```python
from build123d import *

# Parameters (mm, degrees)
SKETCH1_W             = 82.55
SKETCH1_H             = 57.15
BOSS_EXTRUDE1_DEPTH   = 3.175
CUT_EXTRUDE5_DEPTH    = 10
F_8_CLEARANCE_HOLE1_D = 4.4958
F_4_40_TAPPED_HOLE1_D = 2.2606


with BuildPart() as part:
    # Sketch1 → Boss-Extrude1 (new body)
    with BuildSketch(Plane(origin=(0, 0, 0), x_dir=(1, 0, 0), z_dir=(0, 1, 0))):
        Rectangle(SKETCH1_W, SKETCH1_H)
    extrude(amount=BOSS_EXTRUDE1_DEPTH)

    # Sketch2 → Cut-Extrude5 (cut)
    with BuildSketch(Plane.XZ):
        with BuildLine():
            Line((8.5, 1.825), (8.5, 0.175))
            ThreePointArc((8.5, 0.175), (9.42993597, -2.07006403), (11.675, -3))
            Line((11.675, -3), (15.325, -3))
            ThreePointArc((15.325, -3), (17.57006403, -2.07006403), (18.5, 0.175))
            Line((18.5, 0.175), (18.5, 1.825))
            ThreePointArc((18.5, 1.825), (17.57006403, 4.07006403), (15.325, 5))
            Line((15.325, 5), (11.675, 5))
            ThreePointArc((11.675, 5), (9.42993597, 4.07006403), (8.5, 1.825))
        make_face()
    extrude(amount=-CUT_EXTRUDE5_DEPTH, mode=Mode.SUBTRACT)

    # #8 Clearance Hole1 (through all)
    with Locations(Plane(origin=(0, 0, 0), x_dir=(-1, 0, 0), z_dir=(0, -1, 0))):
        with Locations((-37.275, 24.575), (37.275, 24.575), (37.275, -24.575), (-37.275, -24.575)):
            Hole(F_8_CLEARANCE_HOLE1_D / 2)

    # #4-40 Tapped Hole1 (through all)
    with Locations(Plane(origin=(0, 3.175, 0), x_dir=(1, 0, 0), z_dir=(0, 1, 0))):
        with Locations((-29.5, -17), (-29.5, 17), (29.5, 17), (29.5, -17)):
            Hole(F_4_40_TAPPED_HOLE1_D / 2)


solid = part.part
```
Work out the finished part from the listing and answer in its coordinate system (mm). A direction names the side the tool comes from. Round coordinates to 2 decimals unless told otherwise and drop trailing zeros. Write each loop counter-clockwise with the first axis right and the second up, starting at its lowest first coordinate (ties: lowest second). Pieces come first, ordered by that corner, then holes.
1) Determine the mould class of faces 1 (the face through (30.397, 1.565, -16.312)), 2 (the face through (-1, 2, -28.575)), 3 (the face through (41.275, 2, 0)) for opening direction Z: pulls with the +Z half, pulls with the -Z half, needs draft (parallel to the pull), parting line crosses it, or undercut.
2) A cutting plane is placed at B-B on x = -29.5. Determine the outline of the cut face in (y, z) (3 decimals), and give its area (3 significant figures).
3) A cutting plane is placed at D-D on y = 2.6. Give the number of separate pieces and of enclosed holes in the cut face, and give its area (3 significant figures).
4) Consider probe 1 along Z at (x, y) = (-29.5, 1.3) (3 decimals); probe 2 along X at (y, z) = (1.5, 17) (3 decimals); probe 3 along Z at (x, y) = (-37, 2.3) (3 decimals). Determine where each line is inside the solid, lowest interval first.
5) A flat-ended cylindrical pin translates along its axis: P1, Ø3.5, axis at x = 37.275, z = -24.575, coming from the +Y side. Find the tip coordinate at first contact, or state that the pin passes through.
6) A cutting plane is placed at A-A on z = 17. Determine the outline of the cut face in (x, y) (3 decimals), and give its area (3 significant figures).
7) A cutting plane is placed at C-C on z = -2. Determine the outline of the cut face in (x, y) (3 decimals).
8) Which of the six approach directions +Z, -Z, +X, -X, +Y, -Y give full straight-line access (tool end or side, diameter ignored) to faces 4 (the face through (17.55, 1.57, -2.09)), 5 (the face through (-41.275, 2, 0))?
Entries:
1. face 1: undercut
1. face 2: pulls with the -Z half
1. face 3: needs draft
2. outline: (0, -28.575) - (3.175, -28.575) - (3.175, -18.13) - (0, -18.13) - close; (0, -15.87) - (3.175, -15.87) - (3.175, 15.87) - (0, 15.87) - close; (0, 18.13) - (3.175, 18.13) - (3.175, 28.575) - (0, 28.575) - close
2. area: 167 mm2
3. separate pieces: 1
3. enclosed holes: 9
3. area: 4,570 mm2
4. probe 1: z = -28.575 to -18.13, -15.87 to 15.87, 18.13 to 28.575
4. probe 2: x = -41.275 to -30.63, -28.37 to 28.37, 30.63 to 41.275
4. probe 3: z = -28.575 to -26.806, -22.344 to 22.344, 26.806 to 28.575
5. P1: passes through
6. outline: (-41.275, 0) - (-30.63, 0) - (-30.63, 3.175) - (-41.275, 3.175) - close; (-28.37, 0) - (28.37, 0) - (28.37, 3.175) - (-28.37, 3.175) - close; (30.63, 0) - (41.275, 0) - (41.275, 3.175) - (30.63, 3.175) - close
6. area: 248 mm2
7. outline: (-41.275, 0) - (9.362, 0) - (9.362, 3.175) - (-41.275, 3.175) - close; (17.638, 0) - (41.275, 0) - (41.275, 3.175) - (17.638, 3.175) - close
8. face 4: +Y, -Y
8. face 5: +Z, -Z, -X, +Y, -Y
